from build123d import *

# Parameters (mm, degrees)
SKETCH1_R           = 37.5
BOSS_EXTRUDE1_DEPTH = 100
DRAFT1_ANGLE        = 10
SKETCH1_3_W         = 200
SKETCH1_3_H         = 400
BOSS_EXTRUDE2_DEPTH = 150
FILLET1_R           = 59.58768
FILLET2_R           = 25


with BuildPart() as part:
    # Sketch1 → Boss-Extrude1 (new, symmetric)
    with BuildSketch(Plane.YZ):
        Polygon((-900, -100), (-2000, -100), (-2000, 100), (200, 100), (200, -100), (-800, -100), (-800, -275), (-900, -275), align=None)
        with Locations(Location((0, 0, 0), (0, 0, 270))):
            Circle(SKETCH1_R, mode=Mode.SUBTRACT)
    extrude(amount=BOSS_EXTRUDE1_DEPTH, both=True)

    # Draft1
    draft1_faces = [part.faces().sort_by_distance(p)[0] for p in [
        (0, -800, -187.5),
        (0, -900, -187.5),
    ]]
    draft(draft1_faces, Plane(origin=(100, 0, -275), x_dir=(-1, 0, 0), z_dir=(0, 0, -1)), DRAFT1_ANGLE)

    # Sketch1<3> → Boss-Extrude2 (add, symmetric)
    with BuildSketch(Plane.YZ):
        with Locations((-1850, -50)):
            Rectangle(SKETCH1_3_W, SKETCH1_3_H)
    extrude(amount=BOSS_EXTRUDE2_DEPTH, both=True)

    # Fillet1
    fillet1_edges = [part.edges().sort_by_distance(p)[0] for p in [
        (0, -800, -275),
        (0, -900, -275),
    ]]
    fillet(fillet1_edges, radius=FILLET1_R - 0.0001)  # a hair under: the kernel refuses the full size

    # Fillet2
    fillet2_edges = [part.edges().sort_by_distance(p)[0] for p in [
        (0, -769.142778376, -100),
        (0, -930.857221624, -100),
    ]]
    fillet(fillet2_edges, radius=FILLET2_R)


solid = part.part
Read the model definition and answer for the solid it produces. Units are mm, in the model's axes. A direction names the side the tool comes from. Coordinates: 2 decimals unless noted, no trailing zeros. Write each loop counter-clockwise with the first axis right and the second up, starting at its lowest first coordinate (ties: lowest second). Pieces come first, ordered by that corner, then holes. Notation, with made-up numbers: (59, 33) -> (110, 33) arc R18 ccw to (110, 66) -> close; hole circle Ø10 at (38.5, 19.5). An arc over 180 degrees is marked (long way). Return JSON: item names as keys, results as strings.
(1) The part is cut by section C-C on z = 0. Give the vertices of the cut face in (x, y).
Answers below:
{"outline": "(-150, -1950) -> (-100, -1950) -> (-100, -2000) -> (100, -2000) -> (100, -1950) -> (150, -1950) -> (150, -1750) -> (100, -1750) -> (100, -37.5) -> (-100, -37.5) -> (-100, -1750) -> (-150, -1750) -> close; (-100, 37.5) -> (100, 37.5) -> (100, 200) -> (-100, 200) -> close"}
(2) For a pull along Y with two mould halves and no side action, classify faces 4 (the cylindrical face through (1.4, -888.75, -260.68)), 5 (the flat face through (2, -1851, -250)), 6 (the flat face through (1.4, -781.92, -172.47)), 7 (the flat face through (1.4, -917.82, -173.94)) as pulls with the +Y half, pulls with the -Y half, needs draft (parallel to the pull), parting line crosses it, or undercut.
Answers below:
{"face 4": "undercut", "face 5": "needs draft", "face 6": "pulls with the +Y half", "face 7": "undercut"}
(3) Each of these flat-tipped pins is pushed along its axis until it touches: P1, Ø4, axis at x = 5, z = -210.5, coming from the -Y side; P2, Ø3, axis at x = -5, y = -613, coming from the -Z side; P3, Ø12, axis at y = -1687, z = -16, coming from the -X side. Where does it stop, or does it pass through?
Answers below:
{"P1": "y = -1950", "P2": "z = -100", "P3": "x = -100"}
(4) The part is cut by section A-A on y = 0. Give the vertices of the cut face in (x, z), then the cut area to 3 significant figures.
Answers below:
{"outline": "(-100, -100) -> (100, -100) -> (100, -37.5) -> (-100, -37.5) -> close; (-100, 37.5) -> (100, 37.5) -> (100, 100) -> (-100, 100) -> close", "area": "25,000 mm^2"}
(5) Consider line 1 along Y through (x, z) = (-23, 0); line 2 along Y through (x, z) = (133, 86.5); line 3 along Y through (x, z) = (39, -132.5). Determine where each line is inside the solid, lowest interval first. Write a range as from..to.
Answers below:
{"line 1": "-2000..-37.5, 37.5..200", "line 2": "-1950..-1750", "line 3": "-1950..-1750, -925.13..-774.87"}
(6) The part is cut by section D-D on z = -201.5. Give the vertices of the cut face in (x, y).
Answers below:
{"outline": "(-150, -1950) -> (150, -1950) -> (150, -1750) -> (-150, -1750) -> close; (-100, -912.96) -> (100, -912.96) -> (100, -787.04) -> (-100, -787.04) -> close"}
(7) Which of the six approach directions +Z, -Z, +X, -X, +Y, -Y give full straight-line access (tool end or side, diameter ignored) to faces 1 (the flat face through (100, -1975, 1)), 2 (the flat face through (1, -267, -100)), 3 (the flat face through (1, -789, 100))?
Answers below:
{"face 1": "+Z, -Z, +X, -Y", "face 2": "-Z, +X, -X, +Y", "face 3": "+Z, +X, -X, +Y"}
